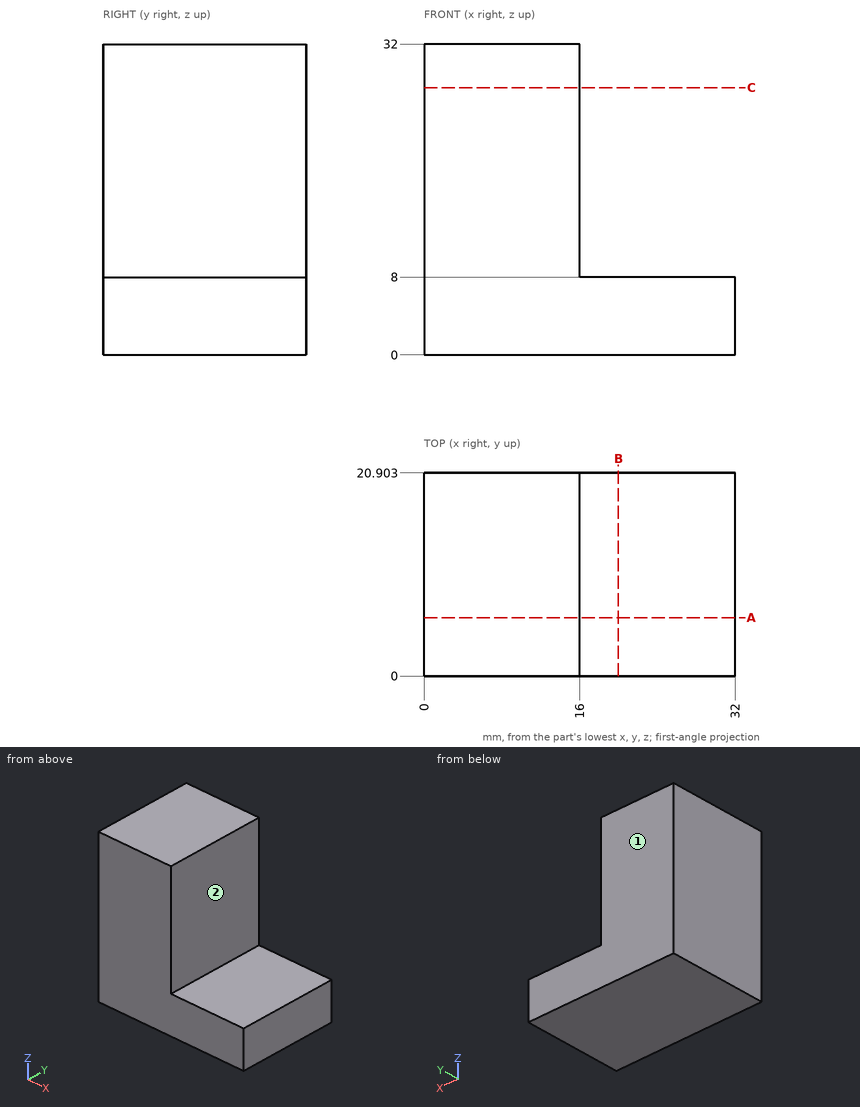
Verification items for this drawing (mm, ordinates from the low corner). A direction names the side the tool comes from. Round coordinates to 2 decimals unless told otherwise and drop trailing zeros. Order: outer loops, then holes, each group sorted by start corner. A loop starts at its lowest first (then second) coordinate and runs counter-clockwise, first axis right, second up. Notation, with made-up numbers: M 4,81 L 12,81 A24 cw 12,119 Z; hole C 88.5,-18.75 d10. An arc over 180 degrees is marked long. Answer in a Markdown table with one row per item. Add a question column.
Item 1: Material ranges on L1, parallel to X at y = 14, z = 20; L2, parallel to Z at x = 25, y = 3, recorded low to high. Write a range as [from, to].
Item 2: Set-up check for the marked faces 1 and 2: record each of +Z, -Z, +X, -X, +Y, -Y from which the full face is reachable in a straight line by a thin tool's end or side.
Item 3: Depth check by flat-ended pin: pin 1 Ø10 at (x, y) = (28.5, 16) entering from +Z. Enter the tip coordinate at first touch or a pass-through.
Item 4: Sectioned sample at B-B, the plane x = 20. Enter the section's corners in (y, z).
Item 5: Sectioned sample at A-A, the plane y = 6. Enter the section's corners in (x, z).
Item 6: Sectioned sample at C-C, the plane z = 27.5. Enter the section's corners in (x, y), plus the area to 3 significant figures.
Filled in:
| question | item | result |
|---|---|---|
| 1 | L1 | x = [0, 16] |
| 1 | L2 | z = [0, 8] |
| 2 | face 1 | +Z, -Z, +X, -X, +Y |
| 2 | face 2 | +Z, +X, +Y, -Y |
| 3 | pin 1 | stops at z = 8 |
| 4 | outline | M 0,0 L 20.9,0 L 20.9,8 L 0,8 Z |
| 5 | outline | M 0,0 L 32,0 L 32,8 L 16,8 L 16,32 L 0,32 Z |
| 6 | outline | M 0,0 L 16,0 L 16,20.9 L 0,20.9 Z |
| 6 | area | 334 mm² |
